Build history of the part. All positions in model axes, mm. A direction names the side the tool comes from. Coordinates: 2 decimals unless noted, no trailing zeros. Order: outer loops, then holes, each group sorted by start corner. A loop starts at its lowest first (then second) coordinate and runs counter-clockwise, first axis right, second up. Notation, with made-up numbers: M 86.5,83.5 L 109.5,83.5 A16 cw 109.5,105.5 Z; hole C 73,32 d7. An arc over 180 degrees is marked long. Use a Markdown table: item, result. Add a question column.
from build123d import *

# Parameters (mm, degrees)
SKETCH_1_R          = 2.5
EXTRUDE_1_DEPTH     = 12
SKETCH_2_R          = 4.75
EXTRUDE_2_DEPTH     = 2.7
FILLET_1_R          = 2
CUT_EXTRUDE_1_DEPTH = 1.56


with BuildPart() as part:
    # 草图1 → 凸台-拉伸1 (new body)
    with BuildSketch(Plane.XY):
        Circle(SKETCH_1_R)
    extrude(amount=EXTRUDE_1_DEPTH)

    # 草图2 → 凸台-拉伸2 (add)
    with BuildSketch(Plane(origin=(0, 0, 0), x_dir=(-1, 0, 0), z_dir=(0, 0, -1))):
        with Locations(Location((0, 0, 0), (0, 0, 180))):
            Circle(SKETCH_2_R)
    extrude(amount=EXTRUDE_2_DEPTH)

    # 圆角1
    fillet_1_edges = [part.edges().sort_by_distance(p)[0] for p in [
        (-4.75, 0, -2.7),
    ]]
    fillet(fillet_1_edges, radius=FILLET_1_R)

    # 草图3 → 切除-拉伸1 (cut)
    with BuildSketch(Plane(origin=(0, 0, -2.7), x_dir=(-1, 0, 0), z_dir=(0, 0, -1))):
        Polygon((1.468584034, 0.918292401), (-0.06097253, 1.730977282), (-1.529556565, 0.812684881), (-1.468584034, -0.918292401), (0.06097253, -1.730977282), (1.529556565, -0.812684881), align=None)
    extrude(amount=-CUT_EXTRUDE_1_DEPTH, mode=Mode.SUBTRACT)


solid = part.part
(1) Drill centre lines: line 1 along Z through (x, y) = (-2.75, -0.5); line 2 along X through (y, z) = (1.5, 4.25); line 3 along X through (y, z) = (-0.5, 7.25). Where is each one in solid material? Low to high. Write a range as from..to.
(2) Drop flat-ended pins along their axis: P1, Ø1.5, axis at x = 1.5, y = -3.5, coming from the +Z side; P2, Ø0.9, axis at x = 0.5, y = -0.5, coming from the -Z side; P3, Ø1, axis at x = -0.5, y = 3.5, coming from the -Z side. Give the stop position or say it passes through.
(3) Slice it at B-B on y = 0. Give the cut face in (x, z).
(4) Slice it at A-A on z = 4.5. Give the cut face in (x, y), and give its area (3 significant figures).
(5) Which spindle directions (+Z, -Z, +X, -X, +Y, -Y) get a long thin tool onto all of the face, cutting with end or side? Do faces 1 (the flat face through (-0.78, -1.28, -1.93)), 2 (the flat face through (0, 0, 12)), 3 (the flat face through (2, 2, 0)). Say none if no direction does.
(6) Mould opens along Y. For faces 4 (the cylindrical face through (-1.03, 4.637, -0.345)), 5 (the flat face through (1.2, 1.2, -2.7)), 6 (the flat face through (0, 0, -1.14)) say: released by +Y, released by -Y, zero draft, split by the parting line, or undercut.
Solutions:
| question | item | result |
|---|---|---|
| 1 | line 1 | -2.7..0 |
| 1 | line 2 | -2..2 |
| 1 | line 3 | -2.45..2.45 |
| 2 | P1 | z = 0 |
| 2 | P2 | z = -1.14 |
| 2 | P3 | z = -2.68 |
| 3 | outline | M -4.75,-0.7 A2 ccw -2.75,-2.7 L -1.5,-2.7 L -1.5,-1.14 L 1.5,-1.14 L 1.5,-2.7 L 2.75,-2.7 A2 ccw 4.75,-0.7 L 4.75,0 L 2.5,0 L 2.5,12 L -2.5,12 L -2.5,0 L -4.75,0 Z |
| 4 | outline | C 0,0 d5 |
| 4 | area | 19.6 mm² |
| 5 | face 1 | -Z |
| 5 | face 2 | +Z, +X, -X, +Y, -Y |
| 5 | face 3 | +Z |
| 6 | face 4 | split by the parting line |
| 6 | face 5 | zero draft |
| 6 | face 6 | undercut |
